Design review of the part built by this model. Coordinates are the model's own, in mm. Face numbers are marked on the shaded views. Round coordinates to 2 decimals unless told otherwise and drop trailing zeros. Write each loop counter-clockwise with the first axis right and the second up, starting at its lowest first coordinate (ties: lowest second). Pieces come first, ordered by that corner, then holes. Notation, with made-up numbers: (41, 34.25) -> (97, 34.25) arc R17 cw to (97, 60.25) -> close; hole circle Ø10 at (43, 52.25). An arc over 180 degrees is marked (long way). Write item = value, one per line. Start each with the question number.
Item 1: Add section A-A, the plane x = 13.5. State the section outline as (y, z) points.
Item 2: Add section B-B, the plane y = 13. State the section outline as (x, z) points, then the cut area to 3 significant figures.
Item 3: Mouldability with a two-part tool opening along X and no side actions: class the marked faces 1, 2, 3 and 4 as released by +X, released by -X, zero draft, split by the parting line, or undercut.
Item 4: Add section C-C, the plane z = 23.5. State the section outline as (x, y) points, then the cut area to 3 significant figures.
Item 5: To check wall thickness, follow L1, parallel to X at y = 6.5, z = 15.25; L2, parallel to X at y = -2, z = 16.5; L3, parallel to Y at x = 10.5, z = 13.25. State the ranges of each line that lie inside material, in increasing order.
from build123d import *

# Parameters (mm, degrees)
F0_W     = 101.6
F0_H     = 76.2
F0_R     = 12.7
F1_DEPTH = 25.4
F2_R     = 3.175
F4_DEPTH = 25.4


with BuildPart() as f1:
    # F0 (on Top) → F1 (new body)
    with BuildSketch(Plane.XY):
        with Locations((7.50792135, 5.9566022065)):
            Rectangle(F0_W, F0_H)
        with Locations((7.50792135, 5.9566022065)):
            Circle(F0_R, mode=Mode.SUBTRACT)
    extrude(amount=F1_DEPTH)

    # F2
    f2_edges = [f1.edges().sort_by_distance(p)[0] for p in [
        (-43.292079, 5.956602, 25.4),
        (7.507921, -32.143398, 25.4),
        (58.307921, 5.956602, 25.4),
        (7.507921, 44.056602, 25.4),
        (-5.192079, 5.956602, 25.4),
        (-43.292079, 5.956602, 0),
        (7.507921, -32.143398, 0),
        (58.307921, 5.956602, 0),
        (7.507921, 44.056602, 0),
        (-5.192079, 5.956602, 0),
        (58.307921, 44.056602, 12.7),
        (-43.292079, 44.056602, 12.7),
        (-43.292079, -32.143398, 12.7),
        (58.307921, -32.143398, 12.7),
    ]]
    fillet(f2_edges, radius=F2_R)


with BuildPart() as f4:
    # F0 (on Top) → F4 (new body)
    with BuildSketch(Plane.XY):
        with Locations((7.50792135, 5.9566022065)):
            Rectangle(F0_W, F0_H)
        with Locations((7.50792135, 5.9566022065)):
            Circle(F0_R, mode=Mode.SUBTRACT)
    extrude(amount=F4_DEPTH)


solid = f4.part
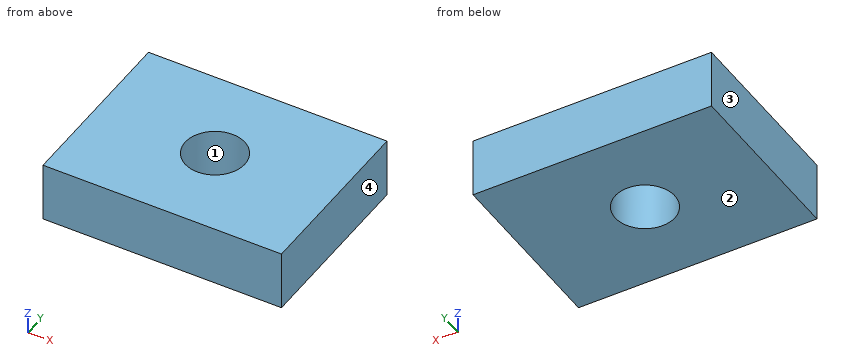
Result set:
q1.outline = (-32.14, 0) -> (-5.24, 0) -> (-5.24, 25.4) -> (-32.14, 25.4) -> close; (17.15, 0) -> (44.06, 0) -> (44.06, 25.4) -> (17.15, 25.4) -> close
q2.outline = (-43.29, 0) -> (-3.06, 0) -> (-3.06, 25.4) -> (-43.29, 25.4) -> close; (18.08, 0) -> (58.31, 0) -> (58.31, 25.4) -> (18.08, 25.4) -> close
q2.area = 2,040 mm²
q3.face_1 = undercut
q3.face_2 = zero draft
q3.face_3 = released by -X
q3.face_4 = released by +X
q4.outline = (-43.29, -32.14) -> (58.31, -32.14) -> (58.31, 44.06) -> (-43.29, 44.06) -> close; hole circle Ø25.4 at (7.51, 5.96)
q4.area = 7,240 mm²
q5.L1 = -43.29 to -5.18, 20.2 to 58.31
q5.L2 = -43.29 to -2.39, 17.41 to 58.31
q5.L3 = -32.14 to -6.39, 18.3 to 44.06
